The model under review builds one solid part; all positions refer to its coordinate system, in mm. Coordinates: 2 decimals unless noted, no trailing zeros. Order: outer loops, then holes, each group sorted by start corner. A loop starts at its lowest first (then second) coordinate and runs counter-clockwise, first axis right, second up. Notation, with made-up numbers: M -26,-33.5 L -12,-33.5 A17 cw -12,-14.5 Z; hole C -3.5,61 d4. An arc over 180 degrees is marked long. One line per item, written item: value.
```python
from build123d import *

# Parameters (mm, degrees)
SKETCH1_R           = 2.5
BOSS_EXTRUDE1_DEPTH = 4


with BuildPart() as part:
    # Sketch1 → Boss-Extrude1 (new body)
    with BuildSketch(Plane.XY):
        with BuildLine():
            Line((0, -122.474747475), (312.5, -122.474747475))
            ThreePointArc((312.5, -122.474747475), (336.217082451, -118.625994829), (357.5, -107.474747475))
            ThreePointArc((357.5, -107.474747475), (425, 27.525252525), (357.5, 162.525252525))
            ThreePointArc((357.5, 162.525252525), (336.217082451, 173.676499879), (312.5, 177.525252525))
            Line((312.5, 177.525252525), (0, 177.525252525))
            Line((0, 177.525252525), (0, 153.525252525))
            Line((0, 153.525252525), (49, 153.525252525))
            Line((49, 153.525252525), (49, -98.474747475))
            Line((49, -98.474747475), (0, -98.474747475))
            Line((0, -98.474747475), (0, -122.474747475))
        make_face()
        with Locations((25, 165.525252525)):
            Circle(SKETCH1_R, mode=Mode.SUBTRACT)
        with Locations((156.25, 165.525252525)):
            Circle(SKETCH1_R, mode=Mode.SUBTRACT)
        with Locations((287.5, 165.525252525)):
            Circle(SKETCH1_R, mode=Mode.SUBTRACT)
        with Locations((332.422349259, 162.292300302)):
            Circle(SKETCH1_R, mode=Mode.SUBTRACT)
        with Locations((395.887987253, 98.741788638)):
            Circle(SKETCH1_R, mode=Mode.SUBTRACT)
        with Locations((413, 27.525252525)):
            Circle(SKETCH1_R, mode=Mode.SUBTRACT)
        with Locations((395.887987253, -43.691283587)):
            Circle(SKETCH1_R, mode=Mode.SUBTRACT)
        with Locations((332.422349259, -107.241795252)):
            Circle(SKETCH1_R, mode=Mode.SUBTRACT)
        with Locations((287.5, -110.474747475)):
            Circle(SKETCH1_R, mode=Mode.SUBTRACT)
        with Locations((156.25, -110.474747475)):
            Circle(SKETCH1_R, mode=Mode.SUBTRACT)
        with Locations((25, -110.474747475)):
            Circle(SKETCH1_R, mode=Mode.SUBTRACT)
    extrude(amount=BOSS_EXTRUDE1_DEPTH)


solid = part.part
```
(1) We need section B-B, the plane z = 3.35. Count the separate pieces of the cut face and the enclosed holes in it, plus the area to 3 significant figures.
Geometry results:
separate pieces: 1
enclosed holes: 11
area: 107,000 mm2
(2) Insertion check: pin 1 Ø1 at (y, z) = (-4, 2) entering from +X; pin 2 Ø4.5 at (x, y) = (287.5, 165.53) entering from -Z; pin 3 Ø2 at (y, z) = (-19, 2) entering from -X. Each pin has a flat end and moves straight along its axis. Give the tip position at first contact, or say it passes through.
Geometry results:
pin 1: stops at x = 422.12
pin 2: passes through
pin 3: stops at x = 49
(3) We need section A-A, the plane x = 34.5. State the section outline as (y, z) points, plus the area to 3 significant figures.
Geometry results:
outline: M -122.47,0 L -98.47,0 L -98.47,4 L -122.47,4 Z; M 153.53,0 L 177.53,0 L 177.53,4 L 153.53,4 Z
area: 192 mm2
(4) For L1, parallel to Y at x = 25, z = 2.1; L2, parallel to Y at x = 287.5, z = 0.95; L3, parallel to Y at x = 43, z = 0.8, list the stretches that pass through material, from the lowest coordinate up.
Geometry results:
L1: y = -122.47 to -112.97, -107.97 to -98.47, 153.53 to 163.03, 168.03 to 177.53
L2: y = -122.47 to -112.97, -107.97 to 163.03, 168.03 to 177.53
L3: y = -122.47 to -98.47, 153.53 to 177.53
(5) We need section D-D, the plane y = 89.5. State the section outline as (x, z) points, plus the area to 3 significant figures.
Geometry results:
outline: M 49,0 L 413.21,0 L 413.21,4 L 49,4 Z
area: 1,460 mm2
(6) We need section C-C, the plane y = 4.5. State the section outline as (x, z) points, plus the area to 3 significant figures.
Geometry results:
outline: M 49,0 L 423.42,0 L 423.42,4 L 49,4 Z
area: 1,500 mm2
